Could you check a few things on this drawing? It's one solid part, dimensions in mm from its lowest x, y, z. A direction names the side the tool comes from. Give positions to 0.01 mm unless a question says otherwise; leave off trailing zeros. Order: outer loops, then holes, each group sorted by start corner. A loop starts at its lowest first (then second) coordinate and runs counter-clockwise, first axis right, second up.
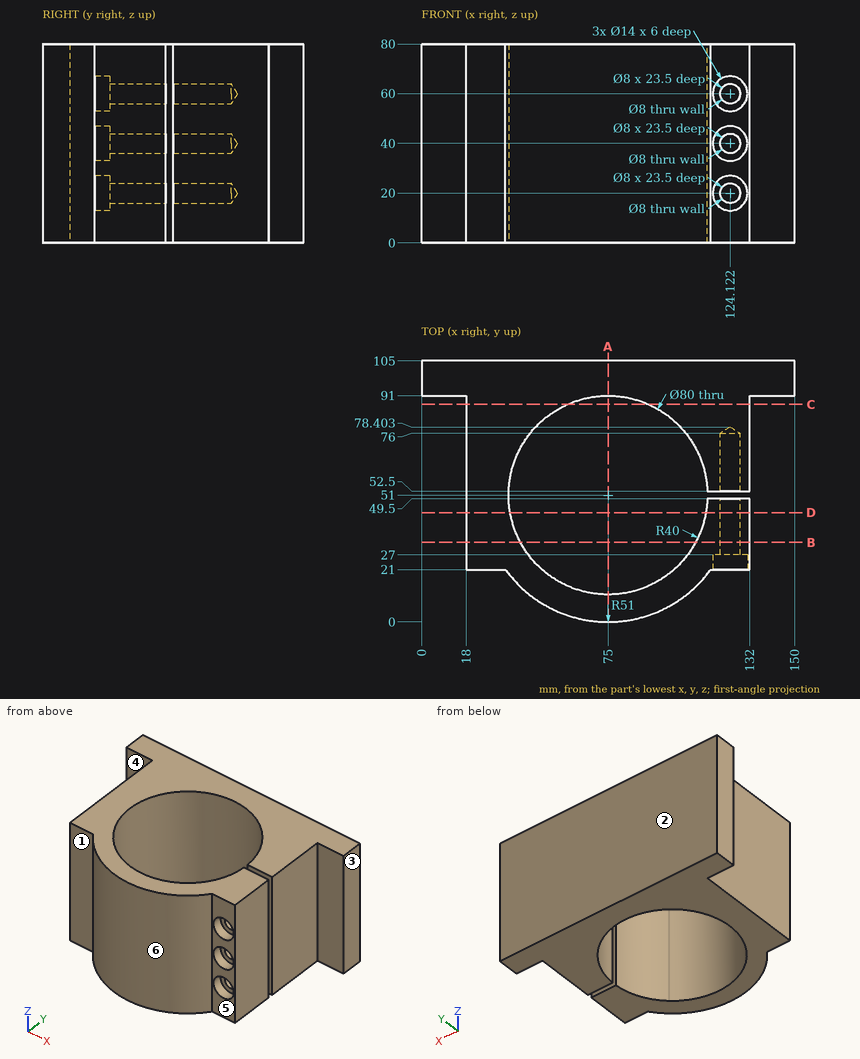
Item 1: Please list where these lines run through material, in increasing order: line 1 along X through (y, z) = (61, 20); line 2 along X through (y, z) = (26, 55) (1 decimal); line 3 along Y through (x, z) = (118, 10).
Findings:
line 1: x = 18 to 36.27, 113.73 to 120.12, 128.12 to 132
line 2: x = 18 to 43.8, 106.2 to 119.2, 129 to 132
line 3: y = 21 to 49.5, 52.5 to 105
Item 2: Imagine slicing it at D-D on y = 44. List the corners of the cut face in (x, z) for me.
Findings:
outline: (18, 0) - (35.62, 0) - (35.62, 80) - (18, 80) - close; (114.38, 0) - (132, 0) - (132, 80) - (114.38, 80) - close; hole circle Ø8 at (124.12, 20); hole circle Ø8 at (124.12, 40); hole circle Ø8 at (124.12, 60)
Item 3: For the marked faces 4, 5 and 6, which set-ups out of +Z, -Z, +X, -X, +Y, -Y let a thin tool reach every point of the face, with its end or its side?
Findings:
face 4: +Z, -Z, -X, -Y
face 5: +Z, -Z, +X, -Y
face 6: +Z, -Z, -Y
Item 4: We'd pull the mould along Y, two halves only. Please class the marked faces 1, 2 and 3: +Y half, -Y half, draft (parallel to the pull), parting line (faces both ways), or undercut.
Findings:
face 1: -Y half
face 2: +Y half
face 3: draft
Item 5: Imagine slicing it at B-B on y = 32. List the corners of the cut face in (x, z) for me.
Findings:
outline: (18, 0) - (39.8, 0) - (39.8, 80) - (18, 80) - close; (110.2, 0) - (132, 0) - (132, 80) - (110.2, 80) - close; hole circle Ø8 at (124.12, 20); hole circle Ø8 at (124.12, 40); hole circle Ø8 at (124.12, 60)
Item 6: Imagine slicing it at C-C on y = 87.5. List the corners of the cut face in (x, z) for me.
Findings:
outline: (18, 0) - (58.64, 0) - (58.64, 80) - (18, 80) - close; (91.36, 0) - (132, 0) - (132, 80) - (91.36, 80) - close
Item 7: Imagine slicing it at A-A on x = 75. List the corners of the cut face in (y, z) for me.
Findings:
outline: (0, 0) - (11, 0) - (11, 80) - (0, 80) - close; (91, 0) - (105, 0) - (105, 80) - (91, 80) - close
Item 8: For pin 1 (22.5 mm diameter, centred on x = 124.12, z = 20, fed in from -Y); pin 2 (1 mm diameter, centred on x = 133, z = 47, fed in from -Y); pin 3 (8 mm diameter, centred on y = 28.5, z = 24, fed in from -X), each with a flat end and sliding along its axis, tell me the tip position at first contact or that it passes through.
Findings:
pin 1: stops at y = 16.84
pin 2: stops at y = 91
pin 3: stops at x = 18
